from build123d import *

# Parameters (mm, degrees)
ESQUISSE1_W                     = 300
ESQUISSE1_H                     = 190
BOSS_EXTRU_1_DEPTH              = 0.5
CHANFREIN1_SIZE                 = 10
CONG_1_R                        = 2
ESQUISSE2_R                     = 2.75
ENL_V_MAT_EXTRU_1_DEPTH         = 1.5
R_P_TITION_LIN_AIRE1_COUNT      = 2
R_P_TITION_LIN_AIRE1_PITCH      = 240
R_P_TITION_LIN_AIRE1_COUNT_DIR2 = 2
R_P_TITION_LIN_AIRE1_PITCH_DIR2 = 160
ESQUISSE4_R                     = 2.75
ESQUISSE4_R_2                   = 20
ESQUISSE4_R_3                   = 15
ENL_V_MAT_EXTRU_3_DEPTH         = 10
ESQUISSE5_R                     = 2.6
ENL_V_MAT_EXTRU_4_DEPTH         = 1.5


with BuildPart() as part:
    # Esquisse1 → Boss.-Extru.1 (new body)
    with BuildSketch(Plane(origin=(0, 0, 0), x_dir=(1, 0, 0), z_dir=(0, 1, 0))):
        Rectangle(ESQUISSE1_W, ESQUISSE1_H)
    extrude(amount=BOSS_EXTRU_1_DEPTH)

    # Chanfrein1
    chanfrein1_edges = [part.edges().sort_by_distance(p)[0] for p in [
        (150, 0.25, 95),
        (-150, 0.25, 95),
        (-150, 0.25, -95),
        (150, 0.25, -95),
    ]]
    chamfer(chanfrein1_edges, length=CHANFREIN1_SIZE)

    # Congé1
    cong_1_edges = [part.edges().sort_by_distance(p)[0] for p in [
        (140, 0.25, 95),
        (-140, 0.25, 95),
        (-150, 0.25, -85),
        (-150, 0.25, 85),
        (150, 0.25, -85),
        (150, 0.25, 85),
        (-140, 0.25, -95),
        (140, 0.25, -95),
    ]]
    fillet(cong_1_edges, radius=CONG_1_R)

    # Esquisse2 → Enlèv. mat.-Extru.1 (cut, through all)
    with BuildSketch(Plane.XZ):
        with Locations((-140, 80)):
            Circle(ESQUISSE2_R)
        with Locations((-100, 80)):
            Circle(ESQUISSE2_R)
    enl_v_mat_extru_1 = extrude(amount=-ENL_V_MAT_EXTRU_1_DEPTH, mode=Mode.SUBTRACT)

    # Répétition linéaire1: Enl_v. mat.-Extru.1 2 × 2
    with Locations(*[(i * R_P_TITION_LIN_AIRE1_PITCH, 0, -j * R_P_TITION_LIN_AIRE1_PITCH_DIR2) for i in range(R_P_TITION_LIN_AIRE1_COUNT) for j in range(R_P_TITION_LIN_AIRE1_COUNT_DIR2) if (i, j) != (0, 0)]):
        add(enl_v_mat_extru_1, mode=Mode.SUBTRACT)

    # Esquisse4 → Enlèv. mat.-Extru.3 (cut)
    with BuildSketch(Plane(origin=(0, 0.5, 0), x_dir=(1, 0, 0), z_dir=(0, 1, 0))):
        with Locations((100, 80)):
            Circle(ESQUISSE4_R)
        with Locations((69.55, 62.8)):
            Circle(ESQUISSE4_R_2)
        Circle(ESQUISSE4_R_3)
    extrude(amount=-ENL_V_MAT_EXTRU_3_DEPTH, mode=Mode.SUBTRACT)

    # Esquisse5 → Enlèv. mat.-Extru.4 (cut, through all)
    with BuildSketch(Plane(origin=(0, 0.5, 0), x_dir=(1, 0, 0), z_dir=(0, 1, 0))):
        with Locations((-30, 30)):
            Circle(ESQUISSE5_R)
        with Locations((30, 30)):
            Circle(ESQUISSE5_R)
        with Locations((30, -30)):
            Circle(ESQUISSE5_R)
        with Locations((-30, -30)):
            Circle(ESQUISSE5_R)
    extrude(amount=-ENL_V_MAT_EXTRU_4_DEPTH, mode=Mode.SUBTRACT)


solid = part.part
Can you work these out from the model? Positions are in its coordinate system, mm. Give positions to 0.01 mm unless a question says otherwise; leave off trailing zeros. Loops run counter-clockwise (first coordinate to the right, second up) from the corner with the lowest first, then second, coordinate; pieces in that order, holes last. Notation, with made-up numbers: M 15.5,-18.5 L 47.5,-18.5 A22 cw 47.5,-11.5 Z; hole C 58,-10 d3. An arc over 180 degrees is marked long. One line per item, written item: value. Start each with the question number.
1) If I drill on line 1 (X direction, y = 0.2, z = -30); line 2 (Z direction, x = -30, y = 0.3); line 3 (Z direction, x = 100, y = 0.35), over which ranges is the centre line in solid material (lowest first)? Write a range as [from, to].
2) If we section it at B-B, the plane x = 69.55: Write out the boundary of the cut face in (y, z), and give its area (3 significant figures).
3) I'm going to push a flat-ended pin straight in: pin 1 (4.5 mm diameter, centred on x = 100, z = 80, fed in from +Y). Where does the tip first touch, or does it pass through?
4) If we section it at A-A, the plane z = -62.8: Write out the boundary of the cut face in (x, y), and give its area (3 significant figures).
5) If we section it at C-C, the plane y = 0.4: Give the number of separate pieces and of enclosed holes in the cut face, and give its area (3 significant figures).
6) Thinking about a two-plate mould opening in X: for faces 1 (the face through (145.1, 0.2, 89.9)), 2 (the face through (142.62, 0.25, -79.17)), 3 (the face through (-144.9, 0.2, -90.1)), 4 (the face through (-2, 0.5, 20)), which applies, +X half, -X half, draft (parallel to the pull), parting line (faces both ways), or undercut?
Completed:
1. line 1: x = [-150, -32.6], [-27.4, 27.4], [32.6, 150]
1. line 2: z = [-95, -32.6], [-27.4, 27.4], [32.6, 95]
1. line 3: z = [-95, -82.75], [-77.25, 77.25], [82.75, 95]
2. outline: M 0,-95 L 0.5,-95 L 0.5,-82.8 L 0,-82.8 Z; M 0,-42.8 L 0.5,-42.8 L 0.5,95 L 0,95 Z
2. area: 75.0 mm^2
3. pin 1: passes through
4. outline: M -150,0 L 49.55,0 L 49.55,0.5 L -150,0.5 Z; M 89.55,0 L 150,0 L 150,0.5 L 89.55,0.5 Z
4. area: 130 mm^2
5. separate pieces: 1
5. enclosed holes: 14
5. area: 54,600 mm^2
6. face 1: +X half
6. face 2: undercut
6. face 3: -X half
6. face 4: draft
